from build123d import *

# Parameters (mm, degrees)
SKETCH_1_W          = 135
SKETCH_1_H          = 75
SKETCH_1_R          = 1.5
SKETCH_1_R_2        = 1.6
EXTRUDE_1_DEPTH     = 2
EXTRUDE_2_DEPTH     = 24
SKETCH_3_R          = 1.5
SKETCH_3_R_2        = 1.6
CUT_EXTRUDE_1_DEPTH = 25


with BuildPart() as part:
    # Эскиз1 → Бобышка-Вытянуть1 (new body)
    with BuildSketch(Plane(origin=(0, 0, 0), x_dir=(1, 0, 0), z_dir=(0, 1, 0))):
        with Locations((67.5, 37.5)):
            Rectangle(SKETCH_1_W, SKETCH_1_H)
        with Locations((3.5, 71)):
            Circle(SKETCH_1_R, mode=Mode.SUBTRACT)
        with Locations((3.5, 35)):
            Circle(SKETCH_1_R_2, mode=Mode.SUBTRACT)
        with Locations((131.5, 71)):
            Circle(SKETCH_1_R, mode=Mode.SUBTRACT)
        with Locations((131.5, 4)):
            Circle(SKETCH_1_R, mode=Mode.SUBTRACT)
    extrude(amount=EXTRUDE_1_DEPTH)

    # Эскиз2 → Бобышка-Вытянуть2 (add)
    with BuildSketch(Plane.XZ):
        Polygon((3.5, -37.886751346), (6, -36.443375673), (6, -33.556624327), (3.5, -32.113248654), (1, -33.556624327), (1, -36.443375673), align=None)
        Polygon((3.5, -73.886751346), (6, -72.443375673), (6, -69.556624327), (3.5, -68.113248654), (1, -69.556624327), (1, -72.443375673), align=None)
        Polygon((131.5, -6.886751346), (134, -5.443375673), (134, -2.556624327), (131.5, -1.113248654), (129, -2.556624327), (129, -5.443375673), align=None)
        Polygon((129, -72.443375673), (131.5, -73.886751346), (134, -72.443375673), (134, -69.556624327), (131.5, -68.113248654), (129, -69.556624327), align=None)
    extrude(amount=EXTRUDE_2_DEPTH)

    # Эскиз3 → Вырез-Вытянуть1 (cut, through all)
    with BuildSketch(Plane(origin=(0, 0, 0), x_dir=(1, 0, 0), z_dir=(0, 1, 0))):
        with Locations((3.5, 71)):
            Circle(SKETCH_3_R)
        with Locations((131.5, 4)):
            Circle(SKETCH_3_R)
        with Locations((131.5, 71)):
            Circle(SKETCH_3_R)
        with Locations((3.5, 35)):
            Circle(SKETCH_3_R_2)
    extrude(amount=-CUT_EXTRUDE_1_DEPTH, mode=Mode.SUBTRACT)


solid = part.part
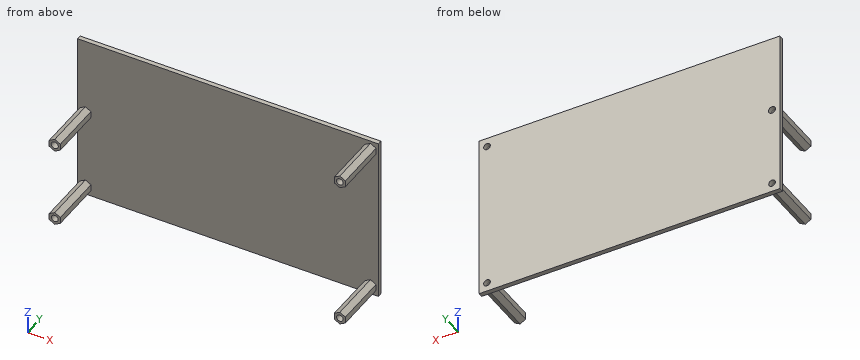
Geometry: final body of the model. Coordinates: model frame, mm. Give positions to 0.01 mm unless a question says otherwise; leave off trailing zeros. Loops run counter-clockwise (first coordinate to the right, second up) from the corner with the lowest first, then second, coordinate; pieces in that order, holes last. Notation, with made-up numbers: (84.5, -7.5) - (138.5, -7.5) arc R17 cw to (138.5, 2.5) - close; hole circle Ø2 at (49.25, 56). An arc over 180 degrees is marked (long way). Answer as CSV lines item,"result". Start each with the question number.
1. Section A-A, the plane y = -13.5. Return loops of the section in (x, z).
2. Section C-C, the plane z = -35. Return loops of the section in (x, y).
3. Ray query, L1, parallel to Z at x = 3.5, y = -13; L2, parallel to Z at x = 3.5, y = 1.25; L3, parallel to Z at x = 131.5, y = 1.1. Return the intervals inside material, ascending.
4. Section D-D, the plane x = 123. Return loops of the section in (y, z), plus the area to 3 significant figures.
5. Section B-B, the plane z = -71. Return loops of the section in (x, y), plus the area to 3 significant figures.
6. Pin query (flat end, axial travel): P1, Ø1.4, axis at y = -16.5, z = -71, coming from the -X side; P2, Ø2.5, axis at x = 131.5, z = -4, coming from the -Y side; P3, Ø1.5, axis at x = 51, z = -29, coming from the -Y side; P4, Ø3, axis at y = -11.5, z = -34.5, coming from the +X side. Return the tip coordinate at first contact, or that it passes through.
Answers:
1,outline,"(1, -72.44) - (3.5, -73.89) - (6, -72.44) - (6, -69.56) - (3.5, -68.11) - (1, -69.56) - close; (1, -36.44) - (3.5, -37.89) - (6, -36.44) - (6, -33.56) - (3.5, -32.11) - (1, -33.56) - close; (129, -72.44) - (131.5, -73.89) - (134, -72.44) - (134, -69.56) - (131.5, -68.11) - (129, -69.56) - close; (129, -5.44) - (131.5, -6.89) - (134, -5.44) - (134, -2.56) - (131.5, -1.11) - (129, -2.56) - close; hole circle Ø3.2 at (3.5, -35); hole circle Ø3 at (3.5, -71); hole circle Ø3 at (131.5, -71); hole circle Ø3 at (131.5, -4)"
2,outline,"(0, 0) - (1, 0) - (1, -24) - (1.9, -24) - (1.9, 2) - (0, 2) - close; (5.1, -24) - (6, -24) - (6, 0) - (135, 0) - (135, 2) - (5.1, 2) - close"
3,L1,"z = -73.89 to -72.5, -69.5 to -68.11, -37.89 to -36.6, -33.4 to -32.11"
3,L2,"z = -75 to -72.5, -69.5 to -36.6, -33.4 to 0"
3,L3,"z = -75 to -72.5, -69.5 to -5.5, -2.5 to 0"
4,outline,"(0, -75) - (2, -75) - (2, 0) - (0, 0) - close"
4,area,"150 mm2"
5,outline,"(0, 0) - (1, 0) - (1, -24) - (2, -24) - (2, 2) - (0, 2) - close; (5, -24) - (6, -24) - (6, 0) - (129, 0) - (129, -24) - (130, -24) - (130, 2) - (5, 2) - close; (133, -24) - (134, -24) - (134, 0) - (135, 0) - (135, 2) - (133, 2) - close"
5,area,"354 mm2"
6,P1,"stops at x = 1"
6,P2,"passes through"
6,P3,"stops at y = 0"
6,P4,"stops at x = 6"
